Input: part model. Units: mm. Frame: model coordinates. Face numbers are marked on the shaded views. A direction names the side the tool comes from. Coordinates: 2 decimals unless noted, no trailing zeros. Loops run counter-clockwise (first coordinate to the right, second up) from the corner with the lowest first, then second, coordinate; pieces in that order, holes last. Notation, with made-up numbers: M 82.25,16 L 119.25,16 A24 ccw 119.25,28 Z; hole C -37,6 d2. An arc over 180 degrees is marked long. Use a Markdown table: item, result. Add a question column.
1. Set-up query: the marked faces 4 and 5. Return all of +Z, -Z, +X, -X, +Y, -Y with unobstructed straight access to the full face (end or side cutting, diameter ignored); none if empty.
2. Section B-B on z = 2. State how many separate pieces and enclosed holes the cut face has, then the cut area to 3 significant figures.
3. Line query: L1, parallel to X at y = 1.5, z = 4; L2, parallel to Y at x = 0.5, z = 3; L3, parallel to Z at x = 13, y = 26. Output: solid intervals per line, ascending. Write a range as [from, to].
4. Section A-A on y = 0. Output: boundary loops of the cut face in (x, z).
5. Draft query along Y for the marked faces 1, 2 and 3. Return one class per face: +Y half, -Y half, draft (parallel to the pull), parting line (faces both ways), or undercut.
6. Pin query (flat end, axial travel): pin 1 (1.7 mm diameter, centred on x = -20, y = -21.5, fed in from -Z); pin 2 (3 mm diameter, centred on x = -20, z = -8.5, fed in from -Y); pin 3 (2 mm diameter, centred on y = -19, z = -4, fed in from -X). Return the tip coordinate at first contact, or that it passes through.
7. Section C-C on x = -14. Output: boundary loops of the cut face in (y, z), then the cut area to 3 significant figures.
```python
from build123d import *

# Parameters (mm, degrees)
SKETCH1_R               = 42.5
BOSS_EXTRUDE1_DEPTH     = 6
SKETCH2_R               = 22
BOSS_EXTRUDE2_DEPTH     = 6
SKETCH3_R               = 20.1
BOSS_EXTRUDE3_DEPTH     = 4.7
SKETCH4_R               = 18.1
CUT_EXTRUDE1_DEPTH      = 11
SKETCH5_R               = 1.75
CUT_EXTRUDE2_DEPTH      = 6.7
SKETCH6_R               = 1.75
CUT_EXTRUDE3_DEPTH      = 12
CUT_EXTRUDE3_DEPTH_BACK = 6.7
SKETCH7_R               = 2.9
CUT_EXTRUDE5_DEPTH      = 3.3
SKETCH8_R               = 1.75
CUT_EXTRUDE6_DEPTH      = 10
SKETCH9_R               = 2.9
CUT_EXTRUDE7_DEPTH      = 3.3


with BuildPart() as part:
    # Sketch1 → Boss-Extrude1 (new body)
    with BuildSketch(Plane.XY):
        Circle(SKETCH1_R)
    extrude(amount=BOSS_EXTRUDE1_DEPTH)

    # Sketch2 → Boss-Extrude2 (add)
    with BuildSketch(Plane(origin=(0, 0, 0), x_dir=(-1, 0, 0), z_dir=(0, 0, -1))):
        Circle(SKETCH2_R)
    extrude(amount=BOSS_EXTRUDE2_DEPTH)

    # Sketch3 → Boss-Extrude3 (add)
    with BuildSketch(Plane(origin=(0, 0, -6), x_dir=(-1, 0, 0), z_dir=(0, 0, -1))):
        Circle(SKETCH3_R)
    extrude(amount=BOSS_EXTRUDE3_DEPTH)

    # Sketch4 → Cut-Extrude1 (cut)
    with BuildSketch(Plane(origin=(0, 0, -10.7), x_dir=(-1, 0, 0), z_dir=(0, 0, -1))):
        Circle(SKETCH4_R)
    extrude(amount=-CUT_EXTRUDE1_DEPTH, mode=Mode.SUBTRACT)

    # Sketch5 → Cut-Extrude2 (cut, through all)
    with BuildSketch(Plane(origin=(0, 0, 0.3), x_dir=(-1, 0, 0), z_dir=(0, 0, -1))):
        with Locations((14, 0)):
            Circle(SKETCH5_R)
        with Locations((0, -14)):
            Circle(SKETCH5_R)
        with Locations((-14, 0)):
            Circle(SKETCH5_R)
        with Locations((0, 14)):
            Circle(SKETCH5_R)
    extrude(amount=-CUT_EXTRUDE2_DEPTH, mode=Mode.SUBTRACT)

    # Sketch6 → Cut-Extrude3 (cut, two sides)
    with BuildSketch(Plane(origin=(0, 0, 0.3), x_dir=(-1, 0, 0), z_dir=(0, 0, -1))) as cut_extrude3_sk:
        with Locations((19.999991423, -20.5)):
            Circle(SKETCH6_R)
        with Locations((-19.999991423, 20.5)):
            Circle(SKETCH6_R)
        with Locations((-19.999991423, -20.5)):
            Circle(SKETCH6_R)
        with Locations((19.999991423, 20.5)):
            Circle(SKETCH6_R)
    extrude(amount=CUT_EXTRUDE3_DEPTH, mode=Mode.SUBTRACT)
    extrude(cut_extrude3_sk.sketch, amount=-CUT_EXTRUDE3_DEPTH_BACK, mode=Mode.SUBTRACT)

    # Sketch7 → Cut-Extrude5 (cut)
    with BuildSketch(Plane.XY):
        with Locations((19.999991423, 20.5)):
            Circle(SKETCH7_R)
        with Locations((-19.999991423, 20.5)):
            Circle(SKETCH7_R)
        with Locations((-19.999991423, -20.5)):
            Circle(SKETCH7_R)
        with Locations((19.999991423, -20.5)):
            Circle(SKETCH7_R)
    extrude(amount=CUT_EXTRUDE5_DEPTH, mode=Mode.SUBTRACT)

    # Sketch8 → Cut-Extrude6 (cut)
    with BuildSketch(Plane.XY.offset(6)):
        with Locations((-29.999991423, -20.5)):
            Circle(SKETCH8_R)
        with Locations((-29.999991423, 20.5)):
            Circle(SKETCH8_R)
        with Locations((29.999991423, 20.5)):
            Circle(SKETCH8_R)
        with Locations((29.999991423, -20.5)):
            Circle(SKETCH8_R)
    extrude(amount=-CUT_EXTRUDE6_DEPTH, mode=Mode.SUBTRACT)

    # Sketch9 → Cut-Extrude7 (cut)
    with BuildSketch(Plane(origin=(0, 0, 0), x_dir=(-1, 0, 0), z_dir=(0, 0, -1))):
        with Locations((-29.999991423, -20.5)):
            Circle(SKETCH9_R)
        with Locations((-29.999991423, 20.5)):
            Circle(SKETCH9_R)
        with Locations((29.999991423, -20.5)):
            Circle(SKETCH9_R)
        with Locations((29.999991423, 20.5)):
            Circle(SKETCH9_R)
    extrude(amount=-CUT_EXTRUDE7_DEPTH, mode=Mode.SUBTRACT)


solid = part.part
```
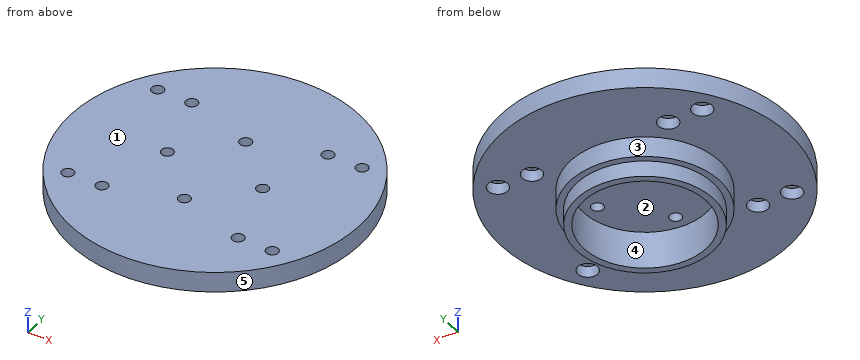
Answers below:
| question | item | result |
|---|---|---|
| 1 | face 4 | -Z |
| 1 | face 5 | +Z, -Z |
| 2 | separate pieces | 1 |
| 2 | enclosed holes | 12 |
| 2 | area | 5,420 mm² |
| 3 | L1 | x = [-42.47, -14.9], [-13.1, 13.1], [14.9, 42.47] |
| 3 | L2 | y = [-42.5, -15.68], [-12.32, 12.32], [15.68, 42.5] |
| 3 | L3 | z = [0, 6] |
| 4 | outline | M -42.5,0 L -22,0 L -22,-6 L -20.1,-6 L -20.1,-10.7 L -18.1,-10.7 L -18.1,0.3 L -15.75,0.3 L -15.75,6 L -42.5,6 Z; M -12.25,0.3 L 12.25,0.3 L 12.25,6 L -12.25,6 Z; M 15.75,0.3 L 18.1,0.3 L 18.1,-10.7 L 20.1,-10.7 L 20.1,-6 L 22,-6 L 22,0 L 42.5,0 L 42.5,6 L 15.75,6 Z |
| 5 | face 1 | draft |
| 5 | face 2 | undercut |
| 5 | face 3 | parting line |
| 6 | pin 1 | stops at z = 3.3 |
| 6 | pin 2 | stops at y = -7.86 |
| 6 | pin 3 | stops at x = -12.65 |
| 7 | outline | M -40.13,0 L -16.97,0 L -16.97,-6 L -14.42,-6 L -14.42,-10.7 L -11.47,-10.7 L -11.47,0.3 L -1.75,0.3 L -1.75,6 L -40.13,6 Z; M 1.75,0.3 L 11.47,0.3 L 11.47,-10.7 L 14.42,-10.7 L 14.42,-6 L 16.97,-6 L 16.97,0 L 40.13,0 L 40.13,6 L 1.75,6 Z |
| 7 | area | 548 mm² |
